Design review of the part built by this model. Coordinates are the model's own, in mm. Face numbers are marked on the shaded views. A direction names the side the tool comes from. Coordinates: 2 decimals unless noted, no trailing zeros. Write each loop counter-clockwise with the first axis right and the second up, starting at its lowest first coordinate (ties: lowest second). Pieces come first, ordered by that corner, then holes. Notation, with made-up numbers: (-38.5, -33) - (-29.5, -33) arc R19 ccw to (-29.5, -3) - close; hole circle Ø2 at (66, 7). An arc over 180 degrees is marked (long way). One line per item, written item: value.
from build123d import *

# Parameters (mm, degrees)
F1_DEPTH = 63.5
F2_DEPTH = 25.4
F3_DEPTH = 7.9375
F0_W     = 25.4
F0_H     = 19.05
F4_DEPTH = 25.4


# Not quite as in the source:
# - a feature names something its author has since deleted; it is built from what else it names


with BuildPart() as f1:
    # F0 (on Front) → F1 (new body, symmetric)
    with BuildSketch(Plane.XZ):
        Polygon((-41.275, 9.525), (-41.275, -9.525), (41.275, -9.525), (41.275, 9.525), (22.225, 9.525), align=None)
    extrude(amount=F1_DEPTH, both=True)

    # F0 (on Front) → F2 (join, symmetric)
    with BuildSketch(Plane.XZ):
        with BuildLine():
            Line((22.225, 9.525), (41.275, 9.525))
            Line((41.275, 9.525), (41.275, 27.0002))
            ThreePointArc((41.275, 27.0002), (45.9246798487, 38.2255201513), (57.15, 42.8752))
            Line((57.15, 42.8752), (60.325, 42.8752))
            Line((60.325, 42.8752), (60.325, 61.9252))
            Line((60.325, 61.9252), (57.15, 61.9252))
            add(Edge.make_bspline(
                [(49.5546191044, 61.0892864361), (52.0673413898, 61.343380394), (54.6014869269, 61.6190974593), (57.15, 61.9252)],
                knots=[0.9527141081, 0.9527141081, 0.9527141081, 0.9527141081, 1, 1, 1, 1], degree=3))
            ThreePointArc((49.5546191044, 61.0892864361), (29.9009238434, 48.8461029022), (22.225, 27.0002))
            Line((22.225, 27.0002), (22.225, 9.525))
        make_face()
    extrude(amount=F2_DEPTH, both=True)

    # F0 (on Front) → F3 (join, symmetric)
    with BuildSketch(Plane.XZ):
        with BuildLine():
            add(Edge.make_bspline(
                [(-41.275, 9.525), (-30.0133153796, 28.1962957233), (-23.3223965861, 57.9111150093), (22.6888247137, 58.3725373278), (49.5546191044, 61.0892864361)],
                knots=[0, 0, 0, 0, 0.4471377236, 0.9527141081, 0.9527141081, 0.9527141081, 0.9527141081], degree=3))
            Line((-41.275, 9.525), (22.225, 9.525))
            Line((22.225, 9.525), (22.225, 27.0002))
            ThreePointArc((22.225, 27.0002), (29.9009238434, 48.8461029022), (49.5546191044, 61.0892864361))
        make_face()
    extrude(amount=F3_DEPTH, both=True)

    # F0 (on Front) → F4 (join, symmetric)
    with BuildSketch(Plane.XZ):
        with Locations((73.025, 52.4002)):
            Rectangle(F0_W, F0_H)
    extrude(amount=F4_DEPTH, both=True)

    # F0 (on Front) → F5 (revolve)
    with BuildSketch(Plane.XZ):
        Polygon((85.725, 66.675), (85.725, 61.9252), (85.725, 42.8752), (85.725, 38.1), (111.125, 38.1), (111.125, 66.675), align=None)
    revolve(axis=Axis((85.725, 0, 52.3875), (0, 0, -1)))


solid = f1.part
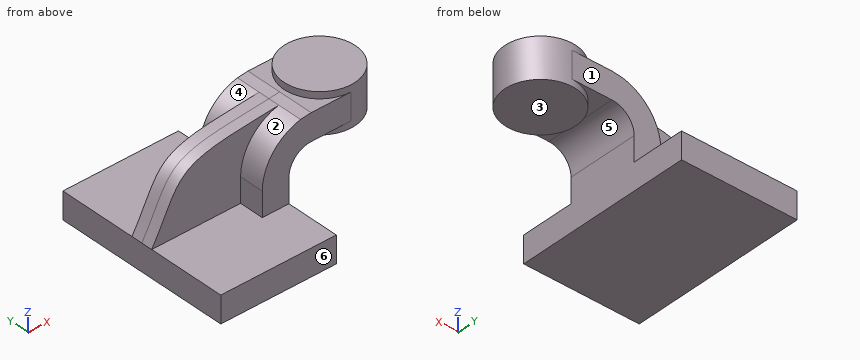
1. Insertion check: pin 1 Ø4 at (x, z) = (79.5, 51.5) entering from -Y; pin 2 Ø1.5 at (x, z) = (8.5, 54.5) entering from +Y; pin 3 Ø1.5 at (x, y) = (60.5, -14) entering from -Z. Each pin has a flat end and moves straight along its axis. Give the tip position at first contact, or say it passes through.
Answer block:
pin 1: stops at y = -25.4
pin 2: stops at y = 7.94
pin 3: stops at z = 42.88
2. Consider section C-C, the plane z = 0. Write out the cut boundary in (x, y) (3 decimals).
Answer block:
outline: (-41.275, -63.5) - (41.275, -63.5) - (41.275, 63.5) - (-41.275, 63.5) - close
3. Mouldability with a two-part tool opening along X and no side actions: class the marked faces 4, 5 and 6 as released by +X, released by -X, zero draft, split by the parting line, or undercut.
Answer block:
face 4: released by -X
face 5: undercut
face 6: zero draft
4. Wall thickness on line 1 along Y through (x, z) = (-2, 43.5); line 2 along Z through (x, y) = (29.5, -40) (3 decimals); line 3 along X through (y, z) = (19, 16) (3 decimals): over which ranges is each line inside the solid? List them lowest first.
Answer block:
line 1: y = -7.94 to 7.94
line 2: z = -9.525 to 9.525
line 3: x = 22.225 to 41.275
5. For the marked faces 1, 2 and 3, list the 3-axis set-ups (+Z, -Z, +X, -X, +Y, -Y) from which the entire face can be reached by the end or side of a thin tool; tool diameter is ignored.
Answer block:
face 1: +Z, +X, -X, +Y
face 2: +Z, -X, -Y
face 3: -Z, +X, +Y, -Y
6. Consider section B-B, the plane y = -34. Write out the cut boundary in (x, z) (3 decimals).
Answer block:
outline: (-41.275, -9.525) - (41.275, -9.525) - (41.275, 9.525) - (-41.275, 9.525) - close
7. Consider section A-A, the plane x = 65. Write out the cut boundary in (y, z) (1 decimal).
Answer block:
outline: (-25.4, 42.9) - (-14.7, 42.9) - (-14.7, 38.1) - (14.7, 38.1) - (14.7, 42.9) - (25.4, 42.9) - (25.4, 61.9) - (14.7, 61.9) - (14.7, 66.7) - (-14.7, 66.7) - (-14.7, 61.9) - (-25.4, 61.9) - close
